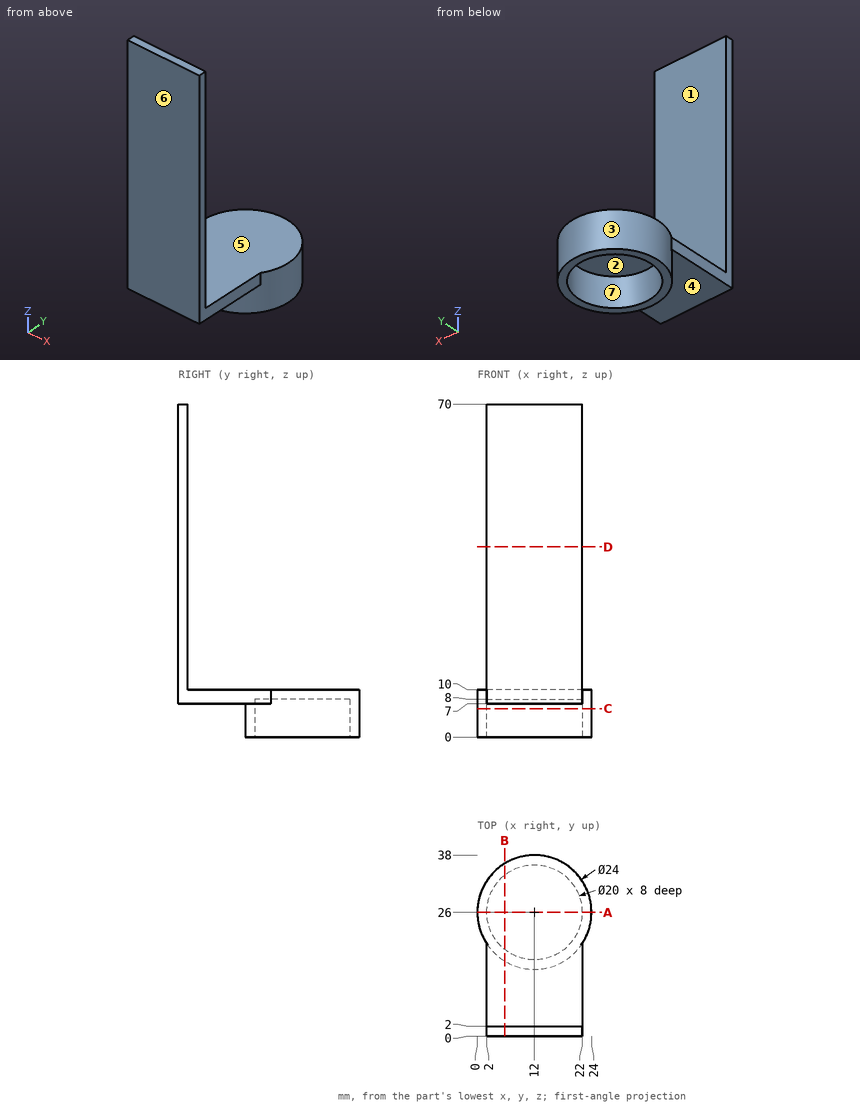
Geometry: see drawing. Coordinates: mm, zero at the bounding-box minimum. A direction names the side the tool comes from. Give positions to 0.01 mm unless a question says otherwise; leave off trailing zeros. Loops run counter-clockwise (first coordinate to the right, second up) from the corner with the lowest first, then second, coordinate; pieces in that order, holes last. Notation, with made-up numbers: (50.25, 33) -> (71.25, 33) arc R20 cw to (71.25, 51) -> close; hole circle Ø8 at (47, -12). An arc over 180 degrees is marked (long way). Use one line per item in the form item = value.
Item 1: Line query: probe 1 along Y at (x, z) = (12, 3.5); probe 2 along Z at (x, y) = (2.25, 23); probe 3 along Y at (x, z) = (6.5, 21). Output: solid intervals per line, ascending.
A:
probe_1 = 14 to 16, 36 to 38
probe_2 = 0 to 10
probe_3 = 0 to 2
Item 2: Section query C-C on z = 6. Output: boundary loops of the cut face in (x, y).
A:
outline = circle Ø24 at (12, 26); hole circle Ø20 at (12, 26)
Item 3: Section query D-D on z = 40. Output: boundary loops of the cut face in (x, y), and give its area (3 significant figures).
A:
outline = (2, 0) -> (22, 0) -> (22, 2) -> (2, 2) -> close
area = 40.0 mm^2
Item 4: Access query for the marked faces 5, 6 and 7. Directions: +Z, -Z, +X, -X, +Y, -Y. A direction counts if a zero-diameter tool reaches every point of the face in a straight line with its end or side. Return the directions, or none.
A:
face_5 = +Z, +X, -X, +Y
face_6 = +Z, -Z, +X, -X, -Y
face_7 = -Z
Item 5: Section query B-B on x = 5.75. Output: boundary loops of the cut face in (y, z).
A:
outline = (0, 7) -> (15.76, 7) -> (15.76, 0) -> (18.19, 0) -> (18.19, 8) -> (33.81, 8) -> (33.81, 0) -> (36.24, 0) -> (36.24, 10) -> (2, 10) -> (2, 70) -> (0, 70) -> close
Item 6: Section query A-A on y = 26. Output: boundary loops of the cut face in (x, z), and give its area (3 significant figures).
A:
outline = (0, 0) -> (2, 0) -> (2, 8) -> (22, 8) -> (22, 0) -> (24, 0) -> (24, 10) -> (0, 10) -> close
area = 80.0 mm^2
Item 7: Draft query along Y for the marked faces 1, 2, 3 and 4. Return one class per face: pulls with the +Y half, pulls with the -Y half, needs draft (parallel to the pull), parting line crosses it, or undercut.
A:
face_1 = pulls with the +Y half
face_2 = undercut
face_3 = parting line crosses it
face_4 = needs draft
Item 8: Pin query (flat end, axial travel): P1, Ø10, axis at x = 17, z = 53.5, coming from the +Y side; P2, Ø12, axis at x = 12, y = 26, coming from the -Z side; P3, Ø21.5, axis at y = 10.5, z = 45.5, coming from the -X side; P4, Ø21.5, axis at y = 14, z = 23, coming from the +X side. Return the tip coordinate at first contact, or that it passes through.
A:
P1 = 2
P2 = 8
P3 = 2
P4 = through
